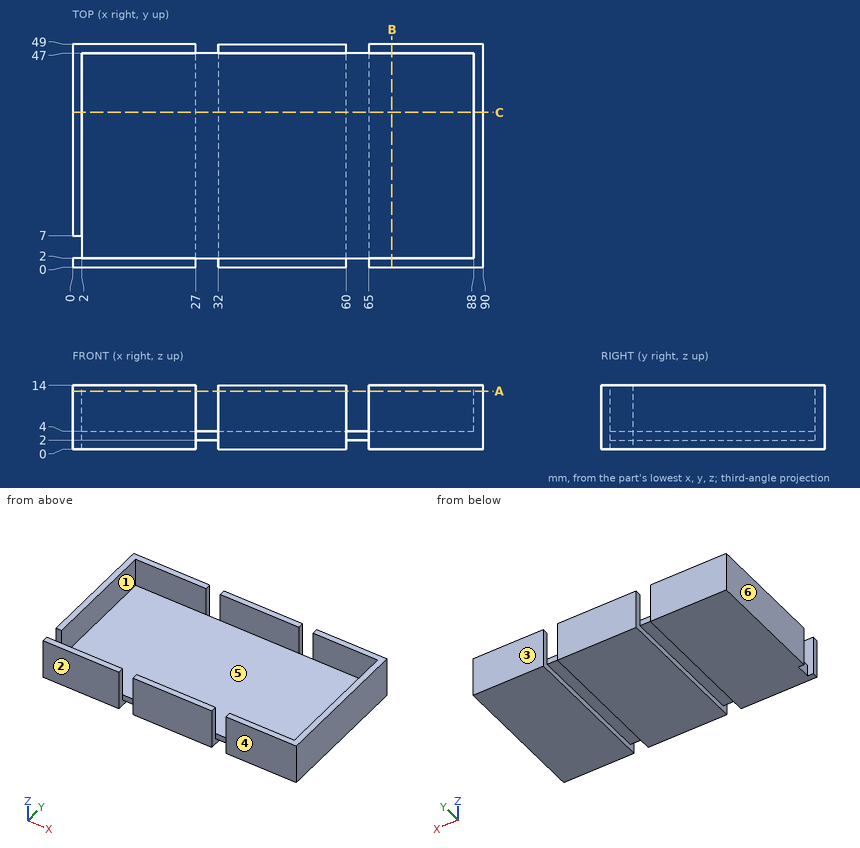
Drawing for the job (mm, zero at the part's lowest x, y, z). A direction names the side the tool comes from. Give positions to 0.01 mm unless a question says otherwise; leave off trailing zeros. Loops run counter-clockwise (first coordinate to the right, second up) from the corner with the lowest first, then second, coordinate; pieces in that order, holes last.
(1) Band-saw the part on C-C (y = 34). Write the cut outline in (x, z), and give its area (3 significant figures).
Return value:
outline: (0, 0) - (27, 0) - (27, 2) - (32, 2) - (32, 0) - (60, 0) - (60, 2) - (65, 2) - (65, 0) - (90, 0) - (90, 14) - (88, 14) - (88, 4) - (2, 4) - (2, 14) - (0, 14) - close
area: 380 mm2
(2) Band-saw the part on B-B (x = 70). Write the cut outline in (y, z).
Return value:
outline: (0, 0) - (49, 0) - (49, 14) - (47, 14) - (47, 4) - (2, 4) - (2, 14) - (0, 14) - close
(3) 3-axis set-ups, long thin cutter, end or side, ignore diameter. For the marked faces 1 and 2: which of +Z, -Z, +X, -X, +Y, -Y reach the whole face in a straight line?
Return value:
face 1: +Z
face 2: +Z, -Z, +X, -X, -Y
(4) Pull direction Y, two halves, no side cores. Call the marked faces 3, 4, 5 and 6: pulls with the +Y half, pulls with the -Y half, needs draft (parallel to the pull), parting line crosses it, or undercut.
Return value:
face 3: pulls with the +Y half
face 4: pulls with the -Y half
face 5: undercut
face 6: needs draft
(5) Pin check, flat tips, straight feed: pin 1 (1.2 mm diameter, centred on y = 3.5, z = 2.5, fed in from -X); pin 2 (2 mm diameter, centred on x = 29.5, z = 3.5, fed in from -Y); pin 3 (4 mm diameter, centred on x = 62.5, y = 29, fed in from -Z). Stop position of each tip, or through.
Return value:
pin 1: stops at x = 2
pin 2: stops at y = 2
pin 3: stops at z = 2
(6) Band-saw the part on A-A (z = 12.75). Write the cut outline in (x, y), and give its area (3 significant figures).
Return value:
outline: (0, 0) - (27, 0) - (27, 2) - (0, 2) - close; (0, 7) - (2, 7) - (2, 47) - (27, 47) - (27, 49) - (0, 49) - close; (32, 0) - (60, 0) - (60, 2) - (32, 2) - close; (32, 47) - (60, 47) - (60, 49) - (32, 49) - close; (65, 0) - (90, 0) - (90, 49) - (65, 49) - (65, 47) - (88, 47) - (88, 2) - (65, 2) - close
area: 490 mm2
(7) Drill centre lines: line 1 along X through (y, z) = (16, 1.5); line 2 along Y through (x, z) = (80.5, 9.25); line 3 along X through (y, z) = (15, 12.25). Where is each one in solid material? Low to high.
Return value:
line 1: x = 0 to 27, 32 to 60, 65 to 90
line 2: y = 0 to 2, 47 to 49
line 3: x = 0 to 2, 88 to 90
